For this review, take the finished solid that the model builds, in its own axes (mm). Face numbers are marked on the shaded views. A direction names the side the tool comes from. Round coordinates to 2 decimals unless told otherwise and drop trailing zeros. Write each loop counter-clockwise with the first axis right and the second up, starting at its lowest first coordinate (ties: lowest second). Pieces come first, ordered by that corner, then holes. Notation, with made-up numbers: M 82.25,67.5 L 110.25,67.5 A32 ccw 110.25,103.5 Z; hole C 2.5,-13 d2. An arc over 180 degrees is marked long. Write each question's results on one line, items separated by ' | '. Start each with the question number.
```python
from build123d import *

# Parameters (mm, degrees)
F0_W      = 152.4
F0_H      = 44.45
F1_DEPTH  = 6.35
F2_W      = 38.1
F2_H      = 30.48
F3_DEPTH  = 12.7
F2_W_2    = 5.08
F2_H_2    = 34.29
F4_DEPTH  = 25.4
F5_R      = 0.508
F6_DEPTH  = 49.2252
F7_SIZE   = 5.08
F8_SIZE   = 1.27
F10_DEPTH = 7.112
F11_W     = 8.2420259714
F11_H     = 14.224
F11_R     = 3.9205193465
F12_DEPTH = 7.874
F13_W     = 2.032
F13_H     = 38.1
F14_DEPTH = 2.032
F15_R     = 0.508
F16_DEPTH = 33.274
F17_W     = 40.4452867806
F17_H     = 44.45
F18_DEPTH = 13.97
F19_W     = 35.2318603545
F19_H     = 10.9959305264
F20_DEPTH = 53.086


with BuildPart() as f1:
    # F0 (on Top) → F1 (new body)
    with BuildSketch(Plane.XY):
        Rectangle(F0_W, F0_H)
    extrude(amount=-F1_DEPTH)

    # F2 (on face) → F3 (join)
    with BuildSketch(Plane(origin=(0, 0, -6.35), x_dir=(1, 0, 0), z_dir=(0, 0, -1))):
        with Locations((29.4156006661, 0)):
            Rectangle(F2_W, F2_H)
    extrude(amount=F3_DEPTH)

    # F2 (on face) → F4 (cut)
    with BuildSketch(Plane(origin=(0, 0, -6.35), x_dir=(1, 0, 0), z_dir=(0, 0, -1))):
        with Locations((73.66, 0)):
            Rectangle(F2_W_2, F2_H_2)
    extrude(amount=-F4_DEPTH, mode=Mode.SUBTRACT)

    # F5 (on face) → F6 (cut)
    with BuildSketch(Plane.XZ.offset(22.225)):
        with Locations((73.7442225218, -3.175)):
            Circle(F5_R)
    extrude(amount=-F6_DEPTH, mode=Mode.SUBTRACT)

    # F7
    f7_edges = [f1.edges().sort_by_distance(p)[0] for p in [
        (10.365601, 0, -19.05),
        (48.465601, 0, -19.05),
    ]]
    chamfer(f7_edges, length=F7_SIZE)

    # F8
    f8_edges = [f1.edges().sort_by_distance(p)[0] for p in [
        (71.12, 0, 0),
        (71.12, 0, -6.35),
    ]]
    chamfer(f8_edges, length=F8_SIZE)

    # F9 (on Front) → F10 (join, symmetric)
    with BuildSketch(Plane.XZ):
        Polygon((-76.2085393071, 0), (-73.0043798685, 0), (-93.789872226, 22.7824151516), (-132.6064432787, 22.7824151516), (-154.8683792353, 0), (-154.8683792353, -11.0822748393), (-146.6263532639, -11.0822748393), (-146.6263532639, -1.9209668972), (-132.6064432787, 13.28467889), (-95.8832409805, 13.28467889), (-76.2085393071, -6.2972982414), align=None)
    extrude(amount=F10_DEPTH, both=True)

    # F11 (on face) → F12 (cut)
    with BuildSketch(Plane(origin=(0, 0, -11.0822748393), x_dir=(1, 0, 0), z_dir=(0, 0, -1))):
        with Locations((-150.7473662496, 0)):
            Rectangle(F11_W, F11_H)
        with Locations((-150.7473662496, 0)):
            Circle(F11_R, mode=Mode.SUBTRACT)
    extrude(amount=-F12_DEPTH, mode=Mode.SUBTRACT)

    # F13 (on face) → F14 (join)
    with BuildSketch(Plane.XY):
        with Locations((-65.9789626062, 0)):
            Rectangle(F13_W, F13_H)
        with Locations((-51.5009626062, 0)):
            Rectangle(F13_W, F13_H)
        with Locations((-37.0229626062, 0)):
            Rectangle(F13_W, F13_H)
        with Locations((-22.5449626062, 0)):
            Rectangle(F13_W, F13_H)
        with Locations((-8.0669626062, 0)):
            Rectangle(F13_W, F13_H)
        with Locations((6.4110373938, 0)):
            Rectangle(F13_W, F13_H)
        with Locations((20.8890373938, 0)):
            Rectangle(F13_W, F13_H)
        with Locations((35.3670373938, 0)):
            Rectangle(F13_W, F13_H)
        with Locations((49.8450373938, 0)):
            Rectangle(F13_W, F13_H)
        with Locations((64.3230373938, 0)):
            Rectangle(F13_W, F13_H)
    extrude(amount=F14_DEPTH)

    # F15 (on face) → F16 (cut)
    with BuildSketch(Plane.XZ.offset(15.24)):
        with Locations((17.9856006661, -16.51)):
            Circle(F15_R)
        with Locations((40.8456006661, -16.51)):
            Circle(F15_R)
    extrude(amount=-F16_DEPTH, mode=Mode.SUBTRACT)

    # F17 (on face) → F18 (join)
    with BuildSketch(Plane(origin=(0, 0, -6.35), x_dir=(1, 0, 0), z_dir=(0, 0, -1))):
        with Locations((-28.8755632937, 0)):
            Rectangle(F17_W, F17_H)
    extrude(amount=F18_DEPTH)

    # F19 (on face) → F20 (cut)
    with BuildSketch(Plane(origin=(0, 22.225, 0), x_dir=(-1, 0, 0), z_dir=(0, 1, 0))):
        with Locations((28.8652880117, -12.0470381808)):
            Rectangle(F19_W, F19_H)
    extrude(amount=-F20_DEPTH, mode=Mode.SUBTRACT)


solid = f1.part
```
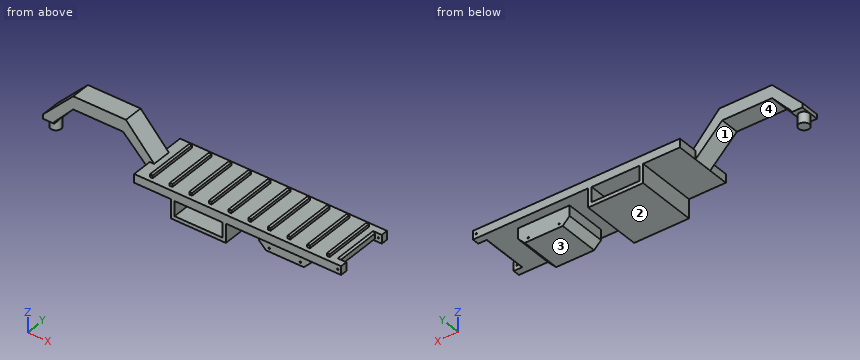
Item 1: For probe 1 along X at (y, z) = (13, -8); probe 2 along X at (y, z) = (1, -6.5); probe 3 along Z at (x, y) = (-47, 4), list the stretches that pass through material, from the lowest coordinate up.
Item 2: Insertion check: P1, Ø0.8, axis at x = 40.85, z = -16.51, coming from the -Y side; P2, Ø6, axis at x = 22, z = -10, coming from the -Y side; P3, Ø1, axis at x = 6.5, z = 1, coming from the +Y side; P4, Ø0.6, axis at x = -51.5, y = -9, coming from the +Z side. Each pin has a flat end and moves straight along its axis. Give the tip position at first contact, or say it passes through.
Item 3: We need section D-D on x = -115.5. State the section outline as (y, z) points.
Item 4: For the marked faces 3 and 4, list the 3-axis set-ups (+Z, -Z, +X, -X, +Y, -Y) from which the entire face can be reached by the end or side of a thin tool; tool diameter is ignored.
Item 5: Mouldability with a two-part tool opening along X and no side actions: class the marked faces 1 and 2 as pulls with the +X half, pulls with the -X half, needs draft (parallel to the pull), parting line crosses it, or undercut.
Item 6: We need section B-B on y = 0. State how many separate pieces and enclosed holes the cut face has, then the cut area to 3 significant figures.
Item 7: We need section C-C on x = 58. State the section outline as (y, z) points (3 decimals), then the cut area to 3 significant figures.
Item 8: We need section A-A on x = -17. State the section outline as (y, z) points (3 decimals), then the cut area to 3 significant figures.
Numbers:
1) probe 1: x = -49.1 to -46.48, -11.25 to -8.65, 10.37 to 48.47 | probe 2: x = -154.54 to -146.96, -49.1 to -8.65, 10.37 to 48.47 | probe 3: z = -20.32 to 0
2) P1: passes through | P2: stops at y = -15.24 | P3: stops at y = 19.05 | P4: stops at z = 2.03
3) outline: M -7.11,13.28 L 7.11,13.28 L 7.11,22.78 L -7.11,22.78 Z
4) face 3: -Z, +X, +Y, -Y | face 4: -Z, +Y, -Y
5) face 1: undercut | face 2: needs draft
6) separate pieces: 1 | enclosed holes: 3 | area: 2,440 mm^2
7) outline: M -22.225,-6.35 L 22.225,-6.35 L 22.225,0 L -22.225,0 Z | area: 282 mm^2
8) outline: M -22.225,-20.32 L 22.225,-20.32 L 22.225,-17.545 L -22.225,-17.545 Z; M -22.225,-6.549 L 22.225,-6.549 L 22.225,0 L -22.225,0 Z | area: 414 mm^2
